Could you check a few things on this model? Use its own coordinates, in mm. Face numbers are marked on the shaded views. Round coordinates to 2 decimals unless told otherwise and drop trailing zeros. Loops run counter-clockwise (first coordinate to the right, second up) from the corner with the lowest first, then second, coordinate; pieces in that order, holes last.
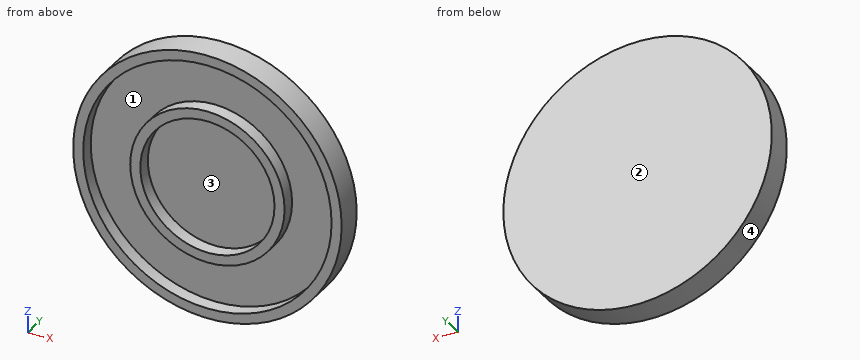
from build123d import *

# Parameters (mm, degrees)
F0_R     = 20
F1_DEPTH = 2
F2_R     = 20
F2_R_2   = 18.5
F3_DEPTH = 2
F4_R     = 11.5
F4_R_2   = 10
F5_DEPTH = 2


with BuildPart() as f1:
    # F0 (on Front) → F1 (new body)
    with BuildSketch(Plane.XZ):
        Circle(F0_R)
    extrude(amount=F1_DEPTH)

    # F2 (on face) → F3 (join)
    with BuildSketch(Plane.XZ.offset(2)):
        Circle(F2_R)
        Circle(F2_R_2, mode=Mode.SUBTRACT)
    extrude(amount=F3_DEPTH)

    # F4 (on face) → F5 (join)
    with BuildSketch(Plane.XZ.offset(2)):
        Circle(F4_R)
        Circle(F4_R_2, mode=Mode.SUBTRACT)
    extrude(amount=F5_DEPTH)


solid = f1.part
Item 1: Will these pins go through, and if not, where does the flat tip stop? pin 1 (4 mm diameter, centred on x = 0, z = 3.5, fed in from -Y); pin 2 (1 mm diameter, centred on x = 14, y = -3.5, fed in from +Z); pin 3 (2 mm diameter, centred on y = -0.5, z = 9, fed in from +X).
Results list:
pin 1: stops at y = -2
pin 2: stops at z = 14.76
pin 3: stops at x = 18.33
Item 2: We'd pull the mould along X, two halves only. Please class the marked faces 1, 2, 3 and 4: released by +X, released by -X, zero draft, split by the parting line, or undercut.
Results list:
face 1: undercut
face 2: zero draft
face 3: undercut
face 4: split by the parting line
Item 3: If we section it at C-C, the plane y = -0.7: Please give me the cut outline in (x, z), then the cut area to 3 significant figures.
Results list:
outline: circle Ø40 at (0, 0)
area: 1,260 mm2
Item 4: If we section it at A-A, the plane z = 0: Please give me the cut outline in (x, y).
Results list:
outline: (-20, -4) - (-18.5, -4) - (-18.5, -2) - (-11.5, -2) - (-11.5, -4) - (-10, -4) - (-10, -2) - (10, -2) - (10, -4) - (11.5, -4) - (11.5, -2) - (18.5, -2) - (18.5, -4) - (20, -4) - (20, 0) - (-20, 0) - close
Item 5: If I drill on line 1 along Z through (x, y) = (0, -2.6); line 2 along Z through (x, y) = (1, -3.55), over which ranges is the centre line in solid material (lowest first)?
Results list:
line 1: z = -20 to -18.5, -11.5 to -10, 10 to 11.5, 18.5 to 20
line 2: z = -19.97 to -18.47, -11.46 to -9.95, 9.95 to 11.46, 18.47 to 19.97
Item 6: If we section it at D-D, the plane x = -17: Please give me the cut outline in (y, z), then the cut area to 3 significant figures.
Results list:
outline: (-4, -10.54) - (0, -10.54) - (0, 10.54) - (-4, 10.54) - (-4, 7.3) - (-2, 7.3) - (-2, -7.3) - (-4, -7.3) - close
area: 55.1 mm2
Item 7: If we section it at B-B, the plane x = 0: Please give me the cut outline in (y, z), then the cut area to 3 significant figures.
Results list:
outline: (-4, -20) - (0, -20) - (0, 20) - (-4, 20) - (-4, 18.5) - (-2, 18.5) - (-2, 11.5) - (-4, 11.5) - (-4, 10) - (-2, 10) - (-2, -10) - (-4, -10) - (-4, -11.5) - (-2, -11.5) - (-2, -18.5) - (-4, -18.5) - close
area: 92.0 mm2
